Input: part model. Units: mm. Frame: model coordinates. Coordinates: 2 decimals unless noted, no trailing zeros. Loops run counter-clockwise (first coordinate to the right, second up) from the corner with the lowest first, then second, coordinate; pieces in that order, holes last.
```python
from build123d import *

# Parameters (mm, degrees)
F1_DEPTH = 6


with BuildPart() as f1:
    # F0 (on Top) → F1 (new body)
    with BuildSketch(Plane.XY):
        with BuildLine():
            ThreePointArc((359.906451, 606), (159.906451, 806), (-40.093549, 606))
            Line((-40.093549, 606), (159.906451, 606))
            Line((159.906451, 606), (159.906451, 600))
            Line((159.906451, 600), (-40.093549, 600))
            Line((-40.093549, 600), (-40.093549, 303))
            Line((-40.093549, 303), (159.906451, 303))
            Line((159.906451, 303), (159.906451, 297))
            Line((159.906451, 297), (-40.093549, 297))
            Line((-40.093549, 297), (-40.093549, 0))
            Line((-40.093549, 0), (159.906451, 0))
            Line((159.906451, 0), (159.906451, -6))
            Line((159.906451, -6), (-40.093549, -6))
            ThreePointArc((-40.093549, -6), (159.906451, -206), (359.906451, -6))
            Line((359.906451, -6), (359.906451, 606))
        make_face()
    extrude(amount=F1_DEPTH)


solid = f1.part
```
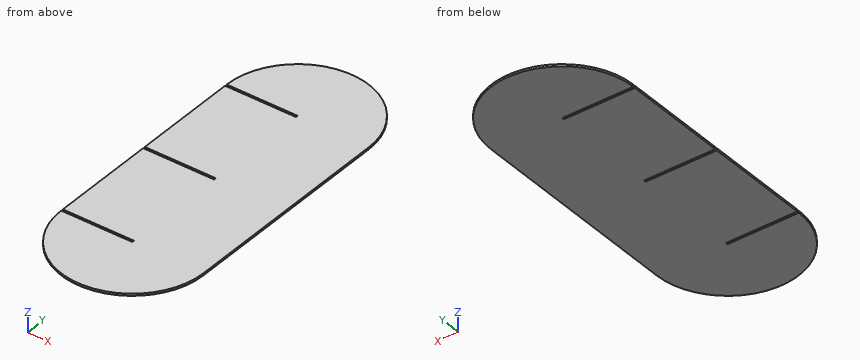
Item 1: Contact query for flat-ended pins moving along their axis: P1, Ø3, axis at y = 621.5, z = 1, coming from the +X side; P2, Ø1.8, axis at x = 29.5, z = 2, coming from the +Y side; P3, Ø2, axis at x = 200, z = 2.5, coming from the -Y side. Output: stop coordinate, or through.
Result:
P1: stops at x = 359.42
P2: stops at y = 758.41
P3: stops at y = -202.14
Item 2: Line query: L1, parallel to Y at x = 84.5, z = 3.85; L2, parallel to Y at x = 35, z = 4.75; L3, parallel to X at y = 613, z = 5.75. Output: solid intervals per line, ascending.
Result:
L1: y = -191.24 to -6, 0 to 297, 303 to 600, 606 to 791.24
L2: y = -162.2 to -6, 0 to 297, 303 to 600, 606 to 762.2
L3: x = -39.97 to 359.78
Item 3: Section query B-B (y = -68). Output: boundary loops of the cut face in (x, z), then the cut area to 3 significant figures.
Result:
outline: (-30.24, 0) - (350.05, 0) - (350.05, 6) - (-30.24, 6) - close
area: 2,280 mm2
Item 4: Section query A-A (z = 1.2). Output: boundary loops of the cut face in (x, y).
Result:
outline: (-40.09, -6) arc R200 ccw to (359.91, -6) - (359.91, 606) arc R200 ccw to (-40.09, 606) - (159.91, 606) - (159.91, 600) - (-40.09, 600) - (-40.09, 303) - (159.91, 303) - (159.91, 297) - (-40.09, 297) - (-40.09, 0) - (159.91, 0) - (159.91, -6) - close
